```python
from build123d import *

# Parameters (mm, degrees)
F1_DEPTH = 1.27
F2_R     = 2.346552
F3_DEPTH = 2.54


with BuildPart() as f1:
    # F0 (on Top) → F1 (new body)
    with BuildSketch(Plane.XY):
        Polygon((12.012586, 46.803898), (0, 46.803898), (-12.012586, 46.803898), (-27.383965, 27.097), (-12.012586, -64.934207), (0, -64.73728), (12.012586, -64.934207), (27.383965, 27.097), align=None)
    extrude(amount=F1_DEPTH)

    # F2 (on face) → F3 (join)
    with BuildSketch(Plane.XY):
        Polygon((0, -62.450973), (10.082072, -62.616252), (24.963741, 26.482971), (10.896499, 44.517897), (0, 44.517897), (-10.896499, 44.517897), (-24.963741, 26.482971), (-10.082072, -62.616252), align=None)
        Polygon((20.66112, 25.391363), (6.650048, -58.495444), (0, -58.386427), (-6.650048, -58.495444), (-20.66112, 25.391363), (-8.912344, 40.453898), (0, 40.453898), (8.912344, 40.453898), align=None, mode=Mode.SUBTRACT)
        Polygon((0, -58.386427), (6.650048, -58.495444), (20.66112, 25.391363), (8.912344, 40.453898), (0, 40.453898), (-8.912344, 40.453898), (-20.66112, 25.391363), (-6.650048, -58.495444), align=None)
        with Locations((0, -53.407203)):
            Circle(F2_R, mode=Mode.SUBTRACT)
    extrude(amount=F3_DEPTH)


solid = f1.part
```
Input: part model. Units: mm. Frame: model coordinates. A direction names the side the tool comes from. Coordinates: 2 decimals unless noted, no trailing zeros. Loops run counter-clockwise (first coordinate to the right, second up) from the corner with the lowest first, then second, coordinate; pieces in that order, holes last.
Q1. Line query: line 1 along Y through (x, z) = (0, 2.2); line 2 along Z through (x, y) = (-16.5, -37.5); line 3 along Y through (x, z) = (-11, 0.55). Output: solid intervals per line, ascending.
Results are:
line 1: y = -62.45 to -55.75, -51.06 to 44.52
line 2: z = 0 to 1.27
line 3: y = -64.92 to 46.8
Q2. Set-up query: faces 1 (the flat face through (-17.627, -17.443, 1.896)), 2 (the flat face through (17.42, -18.69, 1.9)), 3 (the flat face through (-20, -9, 1.27)). Return all of +Z, -Z, +X, -X, +Y, -Y with unobstructed straight access to the full face (end or side cutting, diameter ignored); none if empty.
Results are:
face 1: +Z, -X, -Y
face 2: +Z, +X, -Y
face 3: +Z
Q3. Section C-C, the plane y = 16.5. Return the cut outline in (x, z).
Results are:
outline: (-25.61, 0) - (25.61, 0) - (25.61, 1.27) - (23.3, 1.27) - (23.3, 2.54) - (-23.3, 2.54) - (-23.3, 1.27) - (-25.61, 1.27) - close
Q4. Section B-B, the plane x = -6.5. Return the cut outline in (y, z), and give its area (3 significant figures).
Results are:
outline: (-64.84, 0) - (46.8, 0) - (46.8, 1.27) - (44.52, 1.27) - (44.52, 2.54) - (-62.56, 2.54) - (-62.56, 1.27) - (-64.84, 1.27) - close
area: 278 mm2
Q5. Section A-A, the plane z = 0.75. Return the cut outline in (x, y), and give its area (3 significant figures).
Results are:
outline: (-27.38, 27.1) - (-12.01, -64.93) - (0, -64.74) - (12.01, -64.93) - (27.38, 27.1) - (12.01, 46.8) - (-12.01, 46.8) - close
area: 4,400 mm2
Q6. Mould query, pull axis Y, two halves, no side actions, for faces 4 (the cylindrical face through (-0.31, -51.08, 1.9)), 5 (the flat face through (19.59, -19.56, 0.63)), 6 (the flat face through (-19.59, 37.09, 0.63)). Classes: +Y half, -Y half, draft (parallel to the pull), parting line (faces both ways), or undercut.
Results are:
face 4: undercut
face 5: -Y half
face 6: +Y half
Q7. Contact query for flat-ended pins moving along their axis: pin 1 (1 mm diameter, centred on x = -4.5, z = 2, fed in from +Y); pin 2 (1.5 mm diameter, centred on y = -23.5, z = 1, fed in from +X); pin 3 (2.5 mm diameter, centred on x = 1, y = -53.5, fed in from +Z). Output: stop coordinate, or through.
Results are:
pin 1: stops at y = 44.52
pin 2: stops at x = 19.06
pin 3: stops at z = 1.27
